Part model, mm, in its own coordinate system. A direction names the side the tool comes from. Give positions to 0.01 mm unless a question says otherwise; leave off trailing zeros. Order: outer loops, then holes, each group sorted by start corner. A loop starts at its lowest first (then second) coordinate and runs counter-clockwise, first axis right, second up. Notation, with made-up numbers: M 48.25,70 L 91.25,70 A27 cw 91.25,96 Z; hole C 78,-29.5 d10. An arc over 180 degrees is marked long. Return JSON: item names as keys, results as strings.
from build123d import *

# Parameters (mm, degrees)
SKETCH1_W             = 41.5
SKETCH1_H             = 70
SKETCH1_R             = 1.5
SKETCH1_W_2           = 29.5
SKETCH1_H_2           = 60
BOSS_EXTRUDE1_DEPTH   = 1.143
SKETCH2_W             = 13.25
SKETCH2_H             = 70
BOSS_EXTRUDE2_DEPTH   = 2.286
SKETCH8_W             = 8
SKETCH8_H             = 60
CUT_EXTRUDE1_DEPTH    = 10
SKETCH9_W             = 2.286
SKETCH9_H             = 70
BOSS_EXTRUDE3_DEPTH   = 10.414
F_3_0MM_DOWEL_HOLE1_D = 3


with BuildPart() as part:
    # Sketch1 → Boss-Extrude1 (new body, symmetric)
    with BuildSketch(Plane.XY):
        with Locations((0, 35)):
            Rectangle(SKETCH1_W, SKETCH1_H)
        with Locations((-17.3, 11.25)):
            Circle(SKETCH1_R, mode=Mode.SUBTRACT)
        with Locations((-11, 3.5)):
            Circle(SKETCH1_R, mode=Mode.SUBTRACT)
        with Locations((-17.3, 33.25)):
            Circle(SKETCH1_R, mode=Mode.SUBTRACT)
        with Locations((-17.3, 55.25)):
            Circle(SKETCH1_R, mode=Mode.SUBTRACT)
        with Locations((17.3, 55.25)):
            Circle(SKETCH1_R, mode=Mode.SUBTRACT)
        with Locations((17.3, 33.25)):
            Circle(SKETCH1_R, mode=Mode.SUBTRACT)
        with Locations((11, 3.5)):
            Circle(SKETCH1_R, mode=Mode.SUBTRACT)
        with Locations((17.3, 11.25)):
            Circle(SKETCH1_R, mode=Mode.SUBTRACT)
        with Locations((0, 36)):
            Rectangle(SKETCH1_W_2, SKETCH1_H_2, mode=Mode.SUBTRACT)
    extrude(amount=BOSS_EXTRUDE1_DEPTH, both=True)

    # Sketch2 → Boss-Extrude2 (add)
    with BuildSketch(Plane.XY.offset(1.143)):
        with Locations((-27.375, 35)):
            Rectangle(SKETCH2_W, SKETCH2_H)
    boss_extrude2 = extrude(amount=-BOSS_EXTRUDE2_DEPTH)

    # Mirror4: Boss-Extrude2 across plane
    add(boss_extrude2.mirror(Plane(origin=(0, 0, 0), x_dir=(0, 0, 1), z_dir=(1, 0, 0))))

    # Sketch8 → Cut-Extrude1 (cut)
    with BuildSketch(Plane.XY.offset(1.143)):
        with Locations((-24, 36)):
            Rectangle(SKETCH8_W, SKETCH8_H)
    cut_extrude1 = extrude(amount=-CUT_EXTRUDE1_DEPTH, mode=Mode.SUBTRACT)

    # Mirror3: Cut-Extrude1 across plane
    add(cut_extrude1.mirror(Plane(origin=(0, 0, 0), x_dir=(0, 0, 1), z_dir=(1, 0, 0))), mode=Mode.SUBTRACT)

    # Sketch9 → Boss-Extrude3 (add)
    with BuildSketch(Plane(origin=(0, 0, -1.143), x_dir=(-1, 0, 0), z_dir=(0, 0, -1))):
        with Locations((32.857, 35)):
            Rectangle(SKETCH9_W, SKETCH9_H)
    boss_extrude3 = extrude(amount=BOSS_EXTRUDE3_DEPTH)

    # Mirror5: Boss-Extrude3 across plane
    add(boss_extrude3.mirror(Plane(origin=(0, 0, 0), x_dir=(0, 0, 1), z_dir=(1, 0, 0))))

    # Ø3.0mm Dowel Hole1 (through all)
    with Locations(Plane.ZY.offset(34)):
        with Locations((-6.35, 35), (-6.35, 21), (-6.35, 49), (-6.35, 63), (-6.35, 7)):
            Hole(F_3_0MM_DOWEL_HOLE1_D / 2)


solid = part.part
Q1. Probe line 1 along Y through (x, z) = (32.95, -6.35); line 2 along X through (y, z) = (27, 0.5); line 3 along X through (y, z) = (54, -7.25). List the from-to ranges inside material, lowest first.
Established:
{"line 1": "y = 0 to 5.5, 8.5 to 19.5, 22.5 to 33.5, 36.5 to 47.5, 50.5 to 61.5, 64.5 to 70", "line 2": "x = -34 to -28, -20 to -14.75, 14.75 to 20, 28 to 34", "line 3": "x = -34 to -31.71, 31.71 to 34"}
Q2. 3-axis set-ups, long thin cutter, end or side, ignore diameter. For faces 3 (the flat face through (-14.75, 36, 0)), 4 (the cylindrical face through (-32.841, 64.265, -7.156)), 5 (the flat face through (-31.714, 35, -4)): which of +Z, -Z, +X, -X, +Y, -Y reach the whole face in a straight line?
Established:
{"face 3": "+Z, -Z", "face 4": "+X, -X", "face 5": "-Z, +Y, -Y"}
Q3. Band-saw the part on A-A (y = 42). Give the cut face in (x, z).
Established:
{"outline": "M -34,-11.56 L -31.71,-11.56 L -31.71,-1.14 L -28,-1.14 L -28,1.14 L -34,1.14 Z; M -20,-1.14 L -14.75,-1.14 L -14.75,1.14 L -20,1.14 Z; M 14.75,-1.14 L 20,-1.14 L 20,1.14 L 14.75,1.14 Z; M 28,-1.14 L 31.71,-1.14 L 31.71,-11.56 L 34,-11.56 L 34,1.14 L 28,1.14 Z"}
Q4. Band-saw the part on C-C (z = -2.75). Give the cut face in (x, y), then the cut area to 3 significant figures.
Established:
{"outline": "M -34,0 L -31.71,0 L -31.71,70 L -34,70 Z; M 31.71,0 L 34,0 L 34,70 L 31.71,70 Z", "area": "320 mm²"}
Q5. Two-plate mould, pull along X, no slides. Class faces 1 (the flat face through (0, 66, 0)), 2 (the cylindrical face through (-32.841, 5.536, -6.025)): +X half, -X half, draft (parallel to the pull), parting line (faces both ways), or undercut.
Established:
{"face 1": "undercut", "face 2": "draft"}
Q6. Band-saw the part on D-D (y = 49). Give the cut face in (x, z), then the cut area to 3 significant figures.
Established:
{"outline": "M -34,-11.56 L -31.71,-11.56 L -31.71,-7.85 L -34,-7.85 Z; M -34,-4.85 L -31.71,-4.85 L -31.71,-1.14 L -28,-1.14 L -28,1.14 L -34,1.14 Z; M -20,-1.14 L -14.75,-1.14 L -14.75,1.14 L -20,1.14 Z; M 14.75,-1.14 L 20,-1.14 L 20,1.14 L 14.75,1.14 Z; M 28,-1.14 L 31.71,-1.14 L 31.71,-4.85 L 34,-4.85 L 34,1.14 L 28,1.14 Z; M 31.71,-11.56 L 34,-11.56 L 34,-7.85 L 31.71,-7.85 Z", "area": "85.3 mm²"}
Q7. Pin check, flat tips, straight feed: pin 1 (3.5 mm diameter, centred on x = -17.3, y = 11.25, fed in from -Z); pin 2 (2.5 mm diameter, centred on y = 49, z = -6.35, fed in from +X); pin 3 (4 mm diameter, centred on x = 17.3, y = 55.25, fed in from +Z). Stop position of each tip, or through.
Established:
{"pin 1": "stops at z = -1.14", "pin 2": "passes through", "pin 3": "stops at z = 1.14"}
Q8. Band-saw the part on B-B (x = -22.5). Give the cut face in (y, z).
Established:
{"outline": "M 0,-1.14 L 6,-1.14 L 6,1.14 L 0,1.14 Z; M 66,-1.14 L 70,-1.14 L 70,1.14 L 66,1.14 Z"}
